```python
from build123d import *

# Parameters (mm, degrees)
ESQUISSE1_R        = 6
BOSS_EXTRU_1_DEPTH = 18
CHANFREIN1_SIZE    = 1


with BuildPart() as part:
    # Esquisse1 → Boss.-Extru.1 (new body)
    with BuildSketch(Plane.XY):
        Polygon((9.5, -5.484827557), (9.5, 5.484827557), (0, 10.969655115), (-9.5, 5.484827557), (-9.5, -5.484827557), (0, -10.969655115), align=None)
        Circle(ESQUISSE1_R, mode=Mode.SUBTRACT)
    extrude(amount=BOSS_EXTRU_1_DEPTH)

    # Chanfrein1
    chanfrein1_edges = [part.edges().sort_by_distance(p)[0] for p in [
        (-4.75, -8.227241336, 18),
        (4.75, -8.227241336, 18),
        (9.5, 0, 18),
        (-6, 0, 0),
        (-6, 0, 18),
        (4.75, 8.227241336, 18),
        (-4.75, 8.227241336, 18),
        (4.75, 8.227241336, 0),
        (9.5, 0, 0),
        (4.75, -8.227241336, 0),
        (-9.5, 0, 18),
        (-4.75, -8.227241336, 0),
        (-9.5, 0, 0),
        (-4.75, 8.227241336, 0),
    ]]
    chamfer(chanfrein1_edges, length=CHANFREIN1_SIZE)


solid = part.part
```
Geometry: final body of the model. Coordinates: model frame, mm. Round coordinates to 2 decimals unless told otherwise and drop trailing zeros. Order: outer loops, then holes, each group sorted by start corner. A loop starts at its lowest first (then second) coordinate and runs counter-clockwise, first axis right, second up. Notation, with made-up numbers: (85.5, 59) -> (104.5, 59) arc R30 ccw to (104.5, 95) -> close; hole circle Ø9 at (-26, 28.5). An arc over 180 degrees is marked (long way). Use CSV: the item, a comma, the result in double quotes. Start each with the question number.
1) Material intervals for line 1 along X through (y, z) = (-5.25, 8.75); line 2 along X through (y, z) = (-3, 11.25); line 3 along Y through (x, z) = (-3.25, 13), sorted ascending. Write a range as from..to.
2) First-contact query: pin 1 Ø1.5 at (x, z) = (3.5, 3.5) entering from -Y. Flat tip, straight axial feed; report the tip coordinate or a pass-through.
3) Draft query along X for faces 1 (the face through (-7, 1.5, 0)), 2 (the face through (-6, 0, 9)), 3 (the face through (-4.8, -8.2, 8.9)), 4 (the face through (9, -0.1, 17.5)). Return one class per face: +X half, -X half, draft (parallel to the pull), parting line (faces both ways), or undercut.
4) Section A-A (y = 0). Return the cut outline in (x, z).
5) Section B-B (z = 8.5). Return the cut outline in (x, y), and give its area (3 significant figures).
6) Section C-C (y = 9.5). Return the cut outline in (x, z), and give its area (3 significant figures).
Returned:
1,line 1,"x = -9.5..-2.9, 2.9..9.5"
1,line 2,"x = -9.5..-5.2, 5.2..9.5"
1,line 3,"y = -9.09..-5.04, 5.04..9.09"
2,pin 1,"stops at y = -9.38"
3,face 1,"draft"
3,face 2,"undercut"
3,face 3,"-X half"
3,face 4,"+X half"
4,outline,"(-9.5, 1) -> (-8.5, 0) -> (-7, 0) -> (-6, 1) -> (-6, 17) -> (-7, 18) -> (-8.5, 18) -> (-9.5, 17) -> close; (6, 1) -> (7, 0) -> (8.5, 0) -> (9.5, 1) -> (9.5, 17) -> (8.5, 18) -> (7, 18) -> (6, 17) -> close"
5,outline,"(-9.5, -5.48) -> (0, -10.97) -> (9.5, -5.48) -> (9.5, 5.48) -> (0, 10.97) -> (-9.5, 5.48) -> close; hole circle Ø12 at (0, 0)"
5,area,"200 mm²"
6,outline,"(-2.55, 1) -> (-0.55, 0) -> (0.55, 0) -> (2.55, 1) -> (2.55, 17) -> (0.55, 18) -> (-0.55, 18) -> (-2.55, 17) -> close"
6,area,"87.6 mm²"
